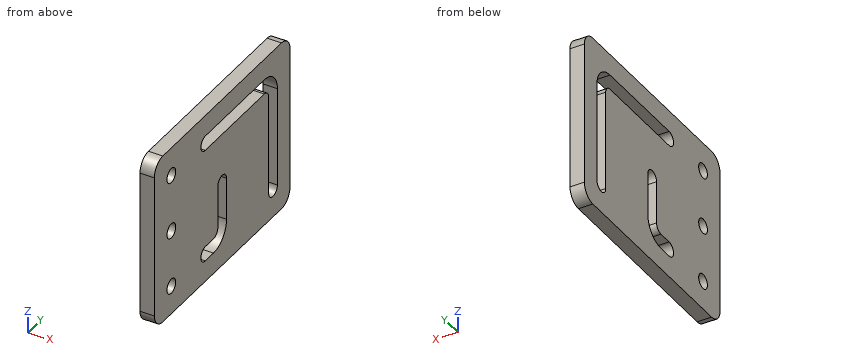
from build123d import *

# Parameters (mm, degrees)
SKETCH1_W      = 76.2
SKETCH1_H      = 101.6
SKETCH1_R      = 3.2639
EXTRUDE1_DEPTH = 6.35
FILLET2_R      = 3.2639
FILLET3_R      = 9.7917
FILLET4_R      = 6.35


with BuildPart() as part:
    # Sketch1 → Extrude1 (new body)
    with BuildSketch(Plane(origin=(0, 0, 0), x_dir=(0, 0, -1), z_dir=(1, 0, 0))):
        with Locations((38.1, 50.8)):
            Rectangle(SKETCH1_W, SKETCH1_H)
        with Locations((12.7, 12.7)):
            Circle(SKETCH1_R, mode=Mode.SUBTRACT)
        with Locations((38.1, 12.7)):
            Circle(SKETCH1_R, mode=Mode.SUBTRACT)
        with Locations((63.5, 12.7)):
            Circle(SKETCH1_R, mode=Mode.SUBTRACT)
        with BuildLine():
            Line((38.1, 47.5361), (60.2361, 47.5361))
            Line((60.2361, 47.5361), (60.2361, 38.1))
            ThreePointArc((60.2361, 38.1), (63.5, 34.8361), (66.7639, 38.1))
            Line((66.7639, 38.1), (66.7639, 54.0639))
            Line((66.7639, 54.0639), (38.1, 54.0639))
            ThreePointArc((38.1, 54.0639), (34.8361, 50.8), (38.1, 47.5361))
        make_face(mode=Mode.SUBTRACT)
        with BuildLine():
            Line((15.9639, 38.1), (15.9639, 85.6361))
            Line((15.9639, 85.6361), (63.5, 85.6361))
            ThreePointArc((63.5, 85.6361), (66.7639, 88.9), (63.5, 92.1639))
            Line((63.5, 92.1639), (9.4361, 92.1639))
            Line((9.4361, 92.1639), (9.4361, 38.1))
            ThreePointArc((9.4361, 38.1), (12.7, 34.8361), (15.9639, 38.1))
        make_face(mode=Mode.SUBTRACT)
    extrude(amount=EXTRUDE1_DEPTH)

    # Fillet2
    fillet2_edges = [part.edges().sort_by_distance(p)[0] for p in [
        (3.175, 47.5361, -60.2361),
        (3.175, 85.6361, -15.9639),
    ]]
    fillet(fillet2_edges, radius=FILLET2_R)

    # Fillet3
    fillet3_edges = [part.edges().sort_by_distance(p)[0] for p in [
        (3.175, 54.0639, -66.7639),
        (3.175, 92.1639, -9.4361),
    ]]
    fillet(fillet3_edges, radius=FILLET3_R)

    # Fillet4
    fillet4_edges = [part.edges().sort_by_distance(p)[0] for p in [
        (3.175, 101.6, 0),
        (3.175, 101.6, -76.2),
        (3.175, 0, -76.2),
        (3.175, 0, 0),
    ]]
    fillet(fillet4_edges, radius=FILLET4_R)


solid = part.part
Geometry check sheet. Reference: the model listing, model coordinates, mm. Give positions to 0.01 mm unless a question says otherwise; leave off trailing zeros. Write each loop counter-clockwise with the first axis right and the second up, starting at its lowest first coordinate (ties: lowest second). Pieces come first, ordered by that corner, then holes. Notation, with made-up numbers: M 71,-11 L 124,-11 A12 ccw 124,-5 Z; hole C 47.5,44 d6. An arc over 180 degrees is marked long. Answer as CSV lines item,"result". Start each with the question number.
Q1. Go/stop test with flat-tipped pins: pin 1 (12 mm diameter, centred on y = 30, z = -45.5, fed in from -X); pin 2 (4 mm diameter, centred on y = 12.7, z = -38.1, fed in from +X). Record where each tip stops, or that it passes through.
Q2. Section check A-A, the plane z = -23. Record the cut outline in (x, y), then the cut area to 3 significant figures.
Q3. Material ranges on L1, parallel to Y at x = 4.75, z = -52.5; L2, parallel to Z at x = 2.5, y = 63.5; L3, parallel to Y at x = 6.25, z = -27, recorded low to high.
Q4. Section check C-C, the plane x = 2.75. Record the cut outline in (y, z), then the cut area to 3 significant figures.
Q5. Section check D-D, the plane y = 56.5. Record the cut outline in (x, z), then the cut area to 3 significant figures.
Q6. Section check B-B, the plane y = 12.7. Record the cut outline in (x, z), then the cut area to 3 significant figures.
Geometry says:
1,pin 1,"x = 0"
1,pin 2,"through"
2,outline,"M 0,0 L 6.35,0 L 6.35,85.64 L 0,85.64 Z; M 0,92.16 L 6.35,92.16 L 6.35,101.6 L 0,101.6 Z"
2,area,"604 mm^2"
3,L1,"0 to 47.54, 54.06 to 85.64, 92.16 to 101.6"
3,L2,"-76.2 to -15.96, -9.44 to 0"
3,L3,"0 to 85.64, 92.16 to 101.6"
4,outline,"M 0,-69.85 A6.35 ccw 6.35,-76.2 L 95.25,-76.2 A6.35 ccw 101.6,-69.85 L 101.6,-6.35 A6.35 ccw 95.25,0 L 6.35,0 A6.35 ccw 0,-6.35 Z; hole C 12.7,-63.5 d6.53; hole C 12.7,-38.1 d6.53; hole C 12.7,-12.7 d6.53; hole M 38.1,-66.76 L 44.27,-66.76 A9.79 ccw 54.06,-56.97 L 54.06,-38.1 A3.26 ccw 47.54,-38.1 L 47.54,-56.97 A3.26 cw 44.27,-60.24 L 38.1,-60.24 A3.26 ccw Z; hole M 38.1,-15.96 L 82.37,-15.96 A3.26 cw 85.64,-19.23 L 85.64,-63.5 A3.26 ccw 92.16,-63.5 L 92.16,-19.23 A9.79 ccw 82.37,-9.44 L 38.1,-9.44 A3.26 ccw Z"
4,area,"6,660 mm^2"
5,outline,"M 0,-76.2 L 6.35,-76.2 L 6.35,-15.96 L 0,-15.96 Z; M 0,-9.44 L 6.35,-9.44 L 6.35,0 L 0,0 Z"
5,area,"442 mm^2"
6,outline,"M 0,-76.2 L 6.35,-76.2 L 6.35,-66.76 L 0,-66.76 Z; M 0,-60.24 L 6.35,-60.24 L 6.35,-41.36 L 0,-41.36 Z; M 0,-34.84 L 6.35,-34.84 L 6.35,-15.96 L 0,-15.96 Z; M 0,-9.44 L 6.35,-9.44 L 6.35,0 L 0,0 Z"
6,area,"360 mm^2"
